from build123d import *

# Parameters (mm, degrees)
SKETCH1_R                 = 7.9375
SKETCH1_R_2               = 3.2639
SKETCH1_R_3               = 1.575
INNER_SIDE_EXTRUDE_DEPTH  = 2.032
OUTER_START               = -9.525
SKETCH1_3_R               = 7.9375
SKETCH1_3_R_2             = 3.2639
SKETCH1_3_R_3             = 1.575
OUTER_SIDE_EXTRUDE_DEPTH  = 9.525
CLEVIS_PIN_CUT_DEPTH      = 15.721869362
CLEVIS_PIN_CUT_DEPTH_BACK = 15.721869362
SKETCH2_R                 = 1.63195
SKETCH3_R                 = 8.255
SKETCH3_R_2               = 7.9375
BOSS_EXTRUDE1_DEPTH       = 4
SKETCH4_R                 = 1.575
CUT_EXTRUDE1_DEPTH        = 4
CHAMFER1_SIZE             = 1
CHAMFER1_SIZE2            = 0.267949192
CUT_EXTRUDE2_DEPTH        = 16.067039421
CUT_EXTRUDE2_DEPTH_BACK   = 16.067039421
SKETCH5_W                 = 16.51
SKETCH5_H                 = 4.312866645


with BuildPart() as part:
    # Sketch1 → Inner Side Extrude (new body)
    with BuildSketch(Plane(origin=(0, 0, 0), x_dir=(0, 0, -1), z_dir=(1, 0, 0))):
        Circle(SKETCH1_R)
        Circle(SKETCH1_R_2, mode=Mode.SUBTRACT)
        with Locations((-5.588, 0)):
            Circle(SKETCH1_R_3, mode=Mode.SUBTRACT)
        with Locations((5.588, 0)):
            Circle(SKETCH1_R_3, mode=Mode.SUBTRACT)
    extrude(amount=INNER_SIDE_EXTRUDE_DEPTH)

    # Sketch1_3 → Outer Side Extrude (add)
    with BuildSketch(Plane(origin=(0, 0, 0), x_dir=(0, 0, -1), z_dir=(1, 0, 0)).offset(OUTER_START)):
        Circle(SKETCH1_3_R)
        Circle(SKETCH1_3_R_2, mode=Mode.SUBTRACT)
        with Locations((-5.588, 0)):
            Circle(SKETCH1_3_R_3, mode=Mode.SUBTRACT)
        with Locations((5.588, 0)):
            Circle(SKETCH1_3_R_3, mode=Mode.SUBTRACT)
    extrude(amount=OUTER_SIDE_EXTRUDE_DEPTH)

    # Sketch2 → Clevis Pin Cut (cut, two sides: drawn at the far end of the back side and taken through both)
    with BuildSketch(Plane(origin=(0, 0, 0), x_dir=(1, 0, 0), z_dir=(0, 1, 0)).offset(-CLEVIS_PIN_CUT_DEPTH_BACK)):
        with Locations(Location((-3.1242, 0, 0), (0, 0, 270))):
            Circle(SKETCH2_R)
    extrude(amount=CLEVIS_PIN_CUT_DEPTH + CLEVIS_PIN_CUT_DEPTH_BACK, mode=Mode.SUBTRACT)

    # Sketch3 → Boss-Extrude1 (add)
    with BuildSketch(Plane(origin=(-9.525, 0, 0), x_dir=(0, 0, -1), z_dir=(1, 0, 0))):
        Circle(SKETCH3_R)
        Circle(SKETCH3_R_2, mode=Mode.SUBTRACT)
    extrude(amount=BOSS_EXTRUDE1_DEPTH)

    # Sketch4 → Cut-Extrude1 (cut)
    # profile 1 of 2: a face of its own
    with BuildSketch(Plane(origin=(-9.525, 0, 0), x_dir=(0, 0, -1), z_dir=(1, 0, 0))):
        Polygon((-3.338, 1.299038106), (-5.588, 2.598076211), (-7.838, 1.299038106), (-7.838, -1.299038106), (-5.588, -2.598076211), (-3.338, -1.299038106), align=None)
        with Locations(Location((-5.588, 0, 0), (0, 0, 180))):
            Circle(SKETCH4_R, mode=Mode.SUBTRACT)
    # profile 2 of 2: a face of its own
    with BuildSketch(Plane(origin=(-9.525, 0, 0), x_dir=(0, 0, -1), z_dir=(1, 0, 0))):
        Polygon((3.338, 1.299038106), (5.588, 2.598076211), (7.838, 1.299038106), (7.838, -1.299038106), (5.588, -2.598076211), (3.338, -1.299038106), align=None)
        with Locations(Location((5.588, 0, 0), (0, 0, 180))):
            Circle(SKETCH4_R, mode=Mode.SUBTRACT)
    extrude(amount=CUT_EXTRUDE1_DEPTH, mode=Mode.SUBTRACT)

    # Chamfer1
    chamfer1_edges = [part.edges().sort_by_distance(p)[0] for p in [
        (-5.525, 0, 8.255),
    ]]
    chamfer1_side = [part.faces().sort_by_distance(p)[0] for p in [
        (-7.525, 0, 8.255),
    ]]
    chamfer(chamfer1_edges, length=CHAMFER1_SIZE, length2=CHAMFER1_SIZE2, reference=chamfer1_side[0])

    # Sketch5 → Cut-Extrude2 (cut, two sides: drawn at the far end of the back side and taken through both)
    with BuildSketch(Plane.XY.offset(-CUT_EXTRUDE2_DEPTH_BACK)):
        with Locations((-3.1242, 7.236433322)):
            Rectangle(SKETCH5_W, SKETCH5_H)
        with Locations((-3.1242, -7.236433322)):
            Rectangle(SKETCH5_W, SKETCH5_H)
    extrude(amount=CUT_EXTRUDE2_DEPTH + CUT_EXTRUDE2_DEPTH_BACK, mode=Mode.SUBTRACT)


solid = part.part
Check sheet for the modelled part. Datum: model origin and axes. Units: mm. A direction names the side the tool comes from. Coordinates: 2 decimals unless noted, no trailing zeros. Loops run counter-clockwise (first coordinate to the right, second up) from the corner with the lowest first, then second, coordinate; pieces in that order, holes last. Notation, with made-up numbers: (5, -21) -> (56, -21) arc R3 ccw to (56, -17) -> close; hole circle Ø6 at (82, 84.5). An arc over 180 degrees is marked (long way). Write item = value, one per line. Start each with the question number.
1. Section check B-B on y = 0. Give the number of separate pieces and of enclosed holes in the cut face, then the cut area to 3 significant figures.
2. Tool access check on faces 4 (the flat face through (-7.55, -1.96, -4.48)), 5 (the flat face through (-5, 5.08, 0)), 6 (the cylindrical face through (-1.799, -0.077, -7.937)). Record the directions out of +Z, -Z, +X, -X, +Y, -Y that give a thin tool (end or side, any length) a straight path to the whole face; none if there is none.
3. Material ranges on line 1 (Y direction, x = -7, z = 0); line 2 (X direction, y = -3.5, z = 0) (3 decimals); line 3 (Z direction, x = -8.25, y = 1.75), recorded low to high.
4. Section check A-A on x = -7.5. Record the cut outline in (y, z) (3 decimals).
5. Draft check along Y on faces 1 (the flat face through (-7.55, 1.94, 4.45)), 2 (the flat face through (-5, -5.08, 0)), 3 (the cylindrical face through (-1.799, 0.077, 7.937)). Enter one of: released by +Y, released by -Y, zero draft, split by the parting line, or undercut.
6. Depth check by flat-ended pin: P1, Ø1.3, axis at y = 0.5, z = -5.5, coming from the -X side. Enter the tip coordinate at first touch or a pass-through.
7. Section check C-C on z = 0. Record the cut outline in (x, y) (3 decimals).
Responses:
q1.separate_pieces = 4
q1.enclosed_holes = 0
q1.area = 26.7 mm2
q2.face_4 = -X
q2.face_5 = +Z, -Z, +X, -X, +Y
q2.face_6 = -Z, +X
q3.line_1 = -5.08 to -3.26, 3.26 to 5.08
q3.line_2 = -9.525 to -4.756, -1.492 to 2.032
q3.line_3 = -8.07 to -7.06, -4.12 to -2.76, 2.76 to 4.12, 7.06 to 8.07
q4.outline = (-5.08, -6.507) arc R8.255 ccw to (5.08, -6.507) -> (5.08, 6.507) arc R8.255 ccw to (-5.08, 6.507) -> close; hole circle Ø6.528 at (0, 0); hole (-2.598, -5.588) -> (-1.299, -7.838) -> (1.299, -7.838) -> (2.598, -5.588) -> (1.299, -3.338) -> (-1.299, -3.338) -> close; hole (-2.598, 5.588) -> (-1.299, 3.338) -> (1.299, 3.338) -> (2.598, 5.588) -> (1.299, 7.838) -> (-1.299, 7.838) -> close
q5.face_1 = undercut
q5.face_2 = released by -Y
q5.face_3 = split by the parting line
q6.P1 = through
q7.outline = (-9.525, -5.08) -> (-4.756, -5.08) -> (-4.756, -3.264) -> (-9.525, -3.264) -> close; (-9.525, 3.264) -> (-4.756, 3.264) -> (-4.756, 5.08) -> (-9.525, 5.08) -> close; (-1.492, -5.08) -> (2.032, -5.08) -> (2.032, -3.264) -> (-1.492, -3.264) -> close; (-1.492, 3.264) -> (2.032, 3.264) -> (2.032, 5.08) -> (-1.492, 5.08) -> close
